from build123d import *

# Parameters (mm, degrees)
F1_DEPTH = 6.35


with BuildPart() as f1:
    # F0 (on Top) → F1 (new body)
    with BuildSketch(Plane.XY):
        with BuildLine():
            Line((0, 0), (0, 19.05))
            Line((0, 19.05), (-6.35, 19.05))
            Line((-6.35, 19.05), (-6.35, 0))
            Line((-6.35, 0), (-19.05, 0))
            Line((-19.05, 0), (-19.05, -6.35))
            Line((-19.05, -6.35), (-9.525, -6.35))
            Line((-9.525, -6.35), (-9.525, -38.1))
            ThreePointArc((-9.525, -38.1), (-7.665128, -42.590128), (-3.175, -44.45))
            ThreePointArc((-3.175, -44.45), (1.315128, -42.590128), (3.175, -38.1))
            Line((3.175, -38.1), (3.175, -6.35))
            Line((3.175, -6.35), (12.7, -6.35))
            Line((12.7, -6.35), (12.7, 0))
            Line((12.7, 0), (0, 0))
        make_face()
    extrude(amount=F1_DEPTH)


solid = f1.part
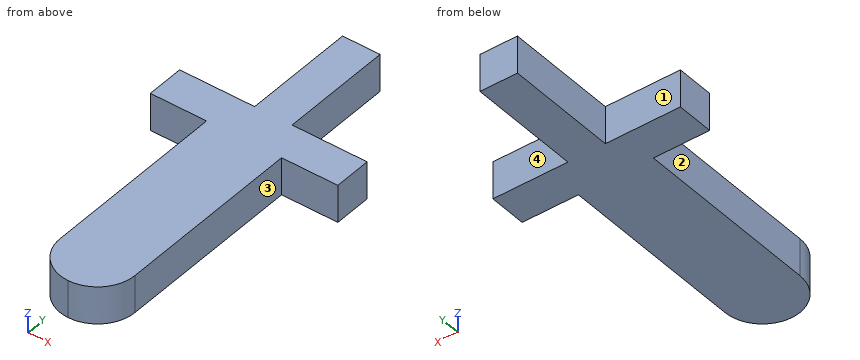
Could you check a few things on this model? Use its own coordinates, in mm. Face numbers are marked on the shaded views. A direction names the side the tool comes from. Give positions to 0.01 mm unless a question says otherwise; leave off trailing zeros. Write each loop counter-clockwise with the first axis right and the second up, starting at its lowest first coordinate (ties: lowest second). Pieces come first, ordered by that corner, then holes. Notation, with made-up numbers: (80, -6.75) - (97, -6.75) arc R16 cw to (97, 1.25) - close; hole circle Ø9 at (49.5, -17). An arc over 180 degrees is marked (long way). Use CSV: the item, a comma, the result in double quotes. Start each with the question number.
Item 1: If I drill on line 1 along Y through (x, z) = (-11, 2); line 2 along X through (y, z) = (-28.5, 3.5) (3 decimals), over which ranges is the centre line in solid material (lowest first)?
Item 2: I'm going to push flat-ended pins straight in: pin 1 (8 mm diameter, centred on x = 6, y = -7, fed in from +Z); pin 2 (3 mm diameter, centred on x = 7.5, z = 4.5, fed in from -Y); pin 3 (1.9 mm diameter, centred on y = 11, z = 4, fed in from -X); pin 4 (1 mm diameter, centred on y = -8.5, z = 5, fed in from -X) (3 decimals). Where does each tip first touch, or does it pass through?
Item 3: I want a section at C-C, the plane y = -28. Please give me the cut outline in (x, z) (3 decimals).
Item 4: I want a section at B-B, the plane x = 4. Please give me the cut outline in (y, z).
Item 5: I want a section at A-A, the plane z = 5.5. Please give me the cut outline in (x, y) (3 decimals), then the cut area to 3 significant figures.
Item 6: For the marked faces 1, 2, 3 and 4, which set-ups out of +Z, -Z, +X, -X, +Y, -Y let a thin tool reach every point of the face, with its end or its side?
Findings:
1,line 1,"y = -6.35 to 0"
1,line 2,"x = -9.525 to 3.175"
2,pin 1,"stops at z = 6.35"
2,pin 2,"stops at y = -6.35"
2,pin 3,"stops at x = -6.35"
2,pin 4,"stops at x = -9.525"
3,outline,"(-9.525, 0) - (3.175, 0) - (3.175, 6.35) - (-9.525, 6.35) - close"
4,outline,"(-6.35, 0) - (0, 0) - (0, 6.35) - (-6.35, 6.35) - close"
5,outline,"(-19.05, -6.35) - (-9.525, -6.35) - (-9.525, -38.1) arc R6.35 ccw to (3.175, -38.1) - (3.175, -6.35) - (12.7, -6.35) - (12.7, 0) - (0, 0) - (0, 19.05) - (-6.35, 19.05) - (-6.35, 0) - (-19.05, 0) - close"
5,area,"789 mm2"
6,face 1,"+Z, -Z, -X, +Y"
6,face 2,"+Z, -Z, -X, -Y"
6,face 3,"+Z, -Z, +X, -Y"
6,face 4,"+Z, -Z, +X, +Y"
